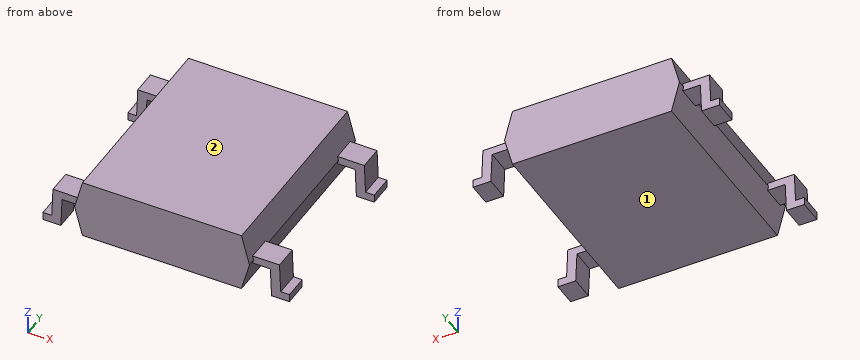
```python
from build123d import *

# Parameters (mm, degrees)
PAD_DEPTH    = 2.5
PAD002_DEPTH = 0.3
PAD001_DEPTH = 0.3


with BuildPart() as pad:
    # Sketch → Pad (new body, symmetric)
    with BuildSketch(Plane.XZ):
        Polygon((-2, 0.1), (2, 0.1), (2.2, 0.85), (2, 1.6), (-2, 1.6), (-2.2, 0.85), align=None)
    extrude(amount=PAD_DEPTH, both=True)


with BuildPart() as pad002:
    # Sketch002 → Pad002 (new body, symmetric)
    with BuildSketch(Plane.XZ.offset(2)):
        Polygon((-3.1, 0), (-2.65, 0), (-2.62, 0.75), (2.62, 0.75), (2.65, 0), (3.1, 0), (3.1, 0.2), (2.88, 0.2), (2.85, 0.95), (-2.85, 0.95), (-2.88, 0.2), (-3.1, 0.2), align=None)
    extrude(amount=PAD002_DEPTH, both=True)


with BuildPart() as obj1:
    # Sketch001 → Pad001 (new body, symmetric)
    with BuildSketch(Plane.XZ.offset(-2)):
        Polygon((-3.1, 0), (-2.65, 0), (-2.62, 0.75), (2.62, 0.75), (2.65, 0), (3.1, 0), (3.1, 0.2), (2.88, 0.2), (2.85, 0.95), (-2.85, 0.95), (-2.88, 0.2), (-3.1, 0.2), align=None)
    extrude(amount=PAD001_DEPTH, both=True)

    add(pad.part)
    add(pad002.part)


solid = obj1.part
```
Could you check a few things on this model? Use its own coordinates, in mm. Face numbers are marked on the shaded views. Round coordinates to 2 decimals unless told otherwise and drop trailing zeros. Write each loop counter-clockwise with the first axis right and the second up, starting at its lowest first coordinate (ties: lowest second). Pieces come first, ordered by that corner, then holes. Notation, with made-up numbers: M 84,21 L 131,21 A24 ccw 131,54 Z; hole C -16.75,-37.5 d9. An arc over 180 degrees is marked long. Write each question's results on one line, items separated by ' | '. Start each with the question number.
1. Imagine slicing it at C-C on x = -1.25. List the corners of the cut face in (y, z) for me, and give its area (3 significant figures).
2. I need wall thicknesses on L1, parallel to Z at x = 0.5, y = -1; L2, parallel to Y at x = -2.25, z = 0.8; L3, parallel to Z at x = 2.25, y = 1.9. Which ranges of each line are inside material? Lowest first, please. Write a range as from..to.
3. I'm going to push flat-ended pins straight in: pin 1 Ø1.5 at (x, y) = (-0.5, 0) entering from -Z; pin 2 Ø0.7 at (x, z) = (2.5, 0.5) entering from -Y; pin 3 Ø0.7 at (x, z) = (2.5, 0.5) entering from +Y. Where does each tip first touch, or does it pass through?
4. Imagine slicing it at D-D on y = -2.05. List the corners of the cut face in (x, z) for me, and give its area (3 significant figures).
5. Imagine slicing it at A-A on z = 0.35. List the corners of the cut face in (x, y) for me, and give its area (3 significant figures).
6. Thinking about a two-plate mould opening in X: for the marked faces 1 and 2, which applies, +X half, -X half, draft (parallel to the pull), parting line (faces both ways), or undercut?
7. Imagine slicing it at B-B on y = -1.5. List the corners of the cut face in (x, z) for me.
Result sheet:
1) outline: M -2.5,0.1 L 2.5,0.1 L 2.5,1.6 L -2.5,1.6 Z | area: 7.50 mm^2
2) L1: z = 0.1..1.6 | L2: y = -2.3..-1.7, 1.7..2.3 | L3: z = 0.75..0.95
3) pin 1: stops at z = 0.1 | pin 2: stops at y = -2.3 | pin 3: stops at y = 2.3
4) outline: M -3.1,0 L -2.65,0 L -2.62,0.75 L -2.17,0.75 L -2,0.1 L 2,0.1 L 2.17,0.75 L 2.62,0.75 L 2.65,0 L 3.1,0 L 3.1,0.2 L 2.88,0.2 L 2.85,0.95 L 2.17,0.95 L 2,1.6 L -2,1.6 L -2.17,0.95 L -2.85,0.95 L -2.88,0.2 L -3.1,0.2 Z | area: 7.01 mm^2
5) outline: M -2.87,-2.3 L -2.64,-2.3 L -2.64,-1.7 L -2.87,-1.7 Z; M -2.87,1.7 L -2.64,1.7 L -2.64,2.3 L -2.87,2.3 Z; M -2.07,-2.5 L 2.07,-2.5 L 2.07,2.5 L -2.07,2.5 Z; M 2.64,-2.3 L 2.87,-2.3 L 2.87,-1.7 L 2.64,-1.7 Z; M 2.64,1.7 L 2.87,1.7 L 2.87,2.3 L 2.64,2.3 Z | area: 21.2 mm^2
6) face 1: undercut | face 2: draft
7) outline: M -2.2,0.85 L -2,0.1 L 2,0.1 L 2.2,0.85 L 2,1.6 L -2,1.6 Z
